```python
from build123d import *

# Parameters (mm, degrees)
F1_DEPTH = 19.05
F3_DEPTH = 6.35


with BuildPart() as f1:
    # F0 (on Right) → F1 (new body)
    with BuildSketch(Plane.YZ):
        Polygon((0, 101.6), (0, 0), (533.4, 0), (533.4, 812.8), (-76.2, 812.8), (-76.2, 101.6), align=None)
    extrude(amount=F1_DEPTH)

    # F2 (on face) → F3 (cut)
    with BuildSketch(Plane(origin=(0, 0, 0), x_dir=(0, -1, 0), z_dir=(-1, 0, 0))):
        Polygon((0, 101.6), (76.2, 101.6), (76.2, 120.65), (-533.4, 120.65), (-533.4, 101.6), align=None)
    extrude(amount=-F3_DEPTH, mode=Mode.SUBTRACT)


solid = f1.part
```
The listing builds one solid part. Answer for the finished solid, in the listing's coordinates (mm). A direction names the side the tool comes from. Give positions to 0.01 mm unless a question says otherwise; leave off trailing zeros. Order: outer loops, then holes, each group sorted by start corner. A loop starts at its lowest first (then second) coordinate and runs counter-clockwise, first axis right, second up.
1) Find section B-B on z = 53. Write down the section's boundary in (x, y).
Reported:
outline: (0, 0) - (19.05, 0) - (19.05, 533.4) - (0, 533.4) - close
2) Consider line 1 along Z through (x, y) = (5, 309); line 2 along Z through (x, y) = (5.75, -18.5); line 3 along Y through (x, z) = (17, 65). Determine where each line is inside the solid, lowest interval first.
Reported:
line 1: z = 0 to 101.6, 120.65 to 812.8
line 2: z = 120.65 to 812.8
line 3: y = 0 to 533.4
3) Find section C-C on y = -33. Write down the section's boundary in (x, z).
Reported:
outline: (0, 120.65) - (6.35, 120.65) - (6.35, 101.6) - (19.05, 101.6) - (19.05, 812.8) - (0, 812.8) - close
4) For faces 1 (the face through (9, -76.2, 462)), 2 (the face through (9, 0, 52)), determine the directions among +Z, -Z, +X, -X, +Y, -Y from which every point of the face is accessible in a straight line to the end or side of a thin tool.
Reported:
face 1: +Z, -Z, +X, -X, -Y
face 2: -Z, +X, -X, -Y
5) Find section A-A on x = 13.5. Write down the section's boundary in (y, z), then the cut area to 3 significant figures.
Reported:
outline: (-76.2, 101.6) - (0, 101.6) - (0, 0) - (533.4, 0) - (533.4, 812.8) - (-76.2, 812.8) - close
area: 488,000 mm2
6) Determine the mould class of faces 3 (the face through (9, 233, 812.8)), 4 (the face through (0, 224, 472)), 5 (the face through (6.35, 233, 111)), 6 (the face through (9, 263, 0)) for opening direction Z: pulls with the +Z half, pulls with the -Z half, needs draft (parallel to the pull), parting line crosses it, or undercut.
Reported:
face 3: pulls with the +Z half
face 4: needs draft
face 5: undercut
face 6: pulls with the -Z half
7) Given P1, Ø4, axis at x = 14, y = -21, coming from the -Z side; P2, Ø5.5, axis at y = 233.5, z = 108.5, coming from the -X side, each flat-ended and moving along its own axis, determine where each tip first touches the part or whether it passes through.
Reported:
P1: stops at z = 101.6
P2: stops at x = 6.35
